```python
from build123d import *

# Parameters (mm, degrees)
BOSS_EXTRUDE1_DEPTH = 0.2


with BuildPart() as part:
    # Sketch1 → Boss-Extrude1 (new body)
    with BuildSketch(Plane(origin=(0, 0, 0), x_dir=(1, 0, 0), z_dir=(0, 1, 0))):
        with BuildLine():
            Line((-19.3, 1.125), (-13.076696831, 1.125))
            ThreePointArc((-13.076696831, 1.125), (0, 13.125), (13.076696831, 1.125))
            Line((13.076696831, 1.125), (19.3, 1.125))
            Line((19.3, 1.125), (19.3, 7.662950904))
            ThreePointArc((19.3, 7.662950904), (19.239103626, 7.969097649), (19.065685426, 8.228636327))
            Line((19.065685426, 8.228636327), (8.366116524, 18.928205229))
            ThreePointArc((8.366116524, 18.928205229), (8.095150585, 19.333734415), (8, 19.812088706))
            Line((8, 19.812088706), (8, 23.124999999))
            Line((8, 23.124999999), (-8, 23.124999999))
            Line((-8, 23.124999999), (-8, 19.812088706))
            ThreePointArc((-8, 19.812088706), (-8.095150585, 19.333734415), (-8.366116524, 18.928205229))
            Line((-8.366116524, 18.928205229), (-19.065685426, 8.228636327))
            ThreePointArc((-19.065685426, 8.228636327), (-19.239103626, 7.969097649), (-19.3, 7.662950904))
            Line((-19.3, 7.662950904), (-19.3, 1.125))
        make_face()
    extrude(amount=-BOSS_EXTRUDE1_DEPTH)


solid = part.part
```
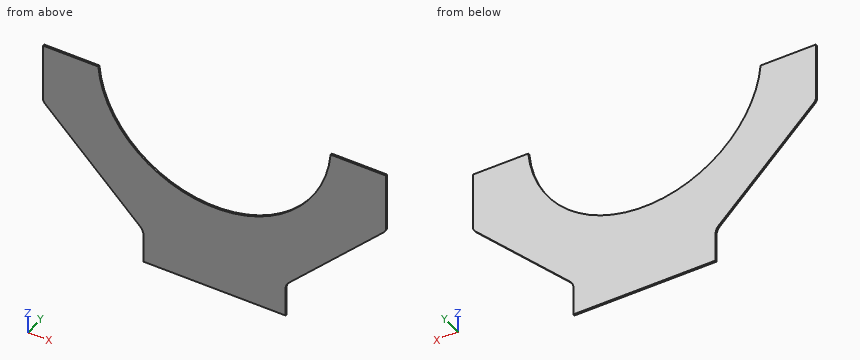
Here's how the part is built. I have some questions about the finished solid (model axes, mm). Coordinates: 2 decimals unless noted, no trailing zeros. Write each loop counter-clockwise with the first axis right and the second up, starting at its lowest first coordinate (ties: lowest second). Pieces come first, ordered by that corner, then holes. Notation, with made-up numbers: (31, 33.5) -> (63, 33.5) arc R22 ccw to (63, 60.5) -> close; hole circle Ø2 at (25, 41.25). An arc over 180 degrees is marked (long way). Use a Markdown table: item, result. Add a question column.
(1) If we section it at D-D, the plane z = -15.5: Write out the boundary of the cut face in (x, y).
(2) If we section it at C-C, the plane x = 0: Write out the boundary of the cut face in (y, z) (3 decimals).
(3) If we section it at A-A, the plane z = -9.5: Write out the boundary of the cut face in (x, y).
(4) If we section it at B-B, the plane y = -0.15: Write out the boundary of the cut face in (x, z) (3 decimals).
(5) Please list where these lines run through material, in increasing order: line 1 (X direction, y = -0.1, z = -21.25); line 2 (X direction, y = -0.05, z = -11.25); line 3 (X direction, y = -0.05, z = -17.75).
Outcome:
| question | item | result |
|---|---|---|
| 1 | outline | (-11.79, -0.2) -> (11.79, -0.2) -> (11.79, 0) -> (-11.79, 0) -> close |
| 2 | outline | (-0.2, -23.125) -> (0, -23.125) -> (0, -13.125) -> (-0.2, -13.125) -> close |
| 3 | outline | (-17.79, -0.2) -> (-9.06, -0.2) -> (-9.06, 0) -> (-17.79, 0) -> close; (9.06, -0.2) -> (17.79, -0.2) -> (17.79, 0) -> (9.06, 0) -> close |
| 4 | outline | (-19.3, -7.663) arc R0.8 ccw to (-19.066, -8.229) -> (-8.366, -18.928) arc R1.25 cw to (-8, -19.812) -> (-8, -23.125) -> (8, -23.125) -> (8, -19.812) arc R1.25 cw to (8.366, -18.928) -> (19.066, -8.229) arc R0.8 ccw to (19.3, -7.663) -> (19.3, -1.125) -> (13.077, -1.125) arc R13.125 cw to (-13.077, -1.125) -> (-19.3, -1.125) -> close |
| 5 | line 1 | x = -8 to 8 |
| 5 | line 2 | x = -16.04 to -6.76, 6.76 to 16.04 |
| 5 | line 3 | x = -9.54 to 9.54 |
